For this review, take the finished solid that the model builds, in its own axes (mm). A direction names the side the tool comes from. Give positions to 0.01 mm unless a question says otherwise; leave off trailing zeros. Order: outer loops, then holes, each group sorted by start corner. A loop starts at its lowest first (then second) coordinate and runs counter-clockwise, first axis right, second up. Notation, with made-up numbers: M 14,8.25 L 43,8.25 A14 ccw 43,24.25 Z; hole C 86,24 d1. An arc over 180 degrees is marked long. Answer as CSV lines item,"result". Start each with the question number.
1. We need section C-C, the plane z = 13. Give the boundary of the cut face in (x, y).
2. Machinability: for faces 4 (the flat face through (-10.3, 20, 46)), 5 (the flat face through (10, 15, 63)), 6 (the flat face through (23, 9, 0)), 7 (the flat face through (0, 0, 11)), 8 (the flat face through (19.5, 9, 63)), which of the approach directions +Z, -Z, +X, -X, +Y, -Y give a long, thin tool a straight path to every point of the face, cutting with its end or side? Answer none if there is none.
3. For line 1 along X through (y, z) = (0.5, 11); line 2 along Z through (x, y) = (12.5, 9.25); line 3 along X through (y, z) = (10, 61), list the stretches that pass through material, from the lowest coordinate up.
4. Clearance check with flat-ended pins moving along their axes: P1, Ø3, axis at y = 12.5, z = 64.5, coming from the +X side; P2, Ø11, axis at y = 14.5, z = 67, coming from the -X side; P3, Ø1, axis at x = -0.5, z = 0.5, coming from the +Y side. State where each tip first meets the part, or that it passes through.
5. We need section D-D, the plane y = 2.5. Give the boundary of the cut face in (x, z), and give its area (3 significant figures).
6. We need section A-A, the plane x = 12.5. Give the boundary of the cut face in (y, z), and give its area (3 significant figures).
7. Mouldability with a two-part tool opening along Z and no side actions: class faces 1 (the flat face through (-19.5, 9, 63)), 2 (the flat face through (-20, 10, 0)), 3 (the flat face through (-21.274, 9.154, 32.86)) as pulls with the +Z half, pulls with the -Z half, needs draft (parallel to the pull), parting line crosses it, or undercut.
8. We need section B-B, the plane y = 11. Give the boundary of the cut face in (x, z), and give its area (3 significant figures).
from build123d import *

# Parameters (mm, degrees)
SKETCH1_W           = 46
SKETCH1_H           = 46
SKETCH1_W_2         = 40
SKETCH1_H_2         = 40
BOSS_EXTRUDE1_DEPTH = 20
SKETCH2_W           = 46
SKETCH2_H           = 46
BOSS_EXTRUDE2_DEPTH = 2
BOSS_EXTRUDE3_DEPTH = 22
CUT_EXTRUDE1_DEPTH  = 20
BOSS_EXTRUDE5_DEPTH = 2
BOSS_EXTRUDE6_DEPTH = 40
SKETCH8_R           = 2.55
CUT_EXTRUDE2_DEPTH  = 60
SKETCH9_W           = 1
SKETCH9_H           = 20
BOSS_EXTRUDE7_DEPTH = 40


with BuildPart() as part:
    # Sketch1 → Boss-Extrude1 (new body)
    with BuildSketch(Plane(origin=(0, 0, 0), x_dir=(1, 0, 0), z_dir=(0, 1, 0))):
        Rectangle(SKETCH1_W, SKETCH1_H)
        Rectangle(SKETCH1_W_2, SKETCH1_H_2, mode=Mode.SUBTRACT)
    extrude(amount=BOSS_EXTRUDE1_DEPTH)

    # Sketch2 → Boss-Extrude2 (add)
    with BuildSketch(Plane.XZ):
        Rectangle(SKETCH2_W, SKETCH2_H)
    extrude(amount=BOSS_EXTRUDE2_DEPTH)

    # Sketch3 → Boss-Extrude3 (add)
    with BuildSketch(Plane(origin=(0, 20, 0), x_dir=(1, 0, 0), z_dir=(0, 1, 0))):
        Polygon((-16, -43), (-19.47826087, -23), (-23, -23), (-19.5, -43), align=None)
        Polygon((23, -23), (19.47826087, -23), (16, -43), (19.5, -43), align=None)
    extrude(amount=-BOSS_EXTRUDE3_DEPTH)

    # Sketch3<3> → Cut-Extrude1 (cut)
    with BuildSketch(Plane(origin=(0, 20, 0), x_dir=(1, 0, 0), z_dir=(0, 1, 0))):
        Polygon((20, -20), (-20, -20), (-19.47826087, -23), (19.47826087, -23), align=None)
    extrude(amount=-CUT_EXTRUDE1_DEPTH, mode=Mode.SUBTRACT)

    # Sketch5 → Boss-Extrude5 (add)
    with BuildSketch(Plane.XZ.offset(2)):
        Polygon((-16, 43), (-19.47826087, 23), (19.47826087, 23), (16, 43), align=None)
    extrude(amount=-BOSS_EXTRUDE5_DEPTH)

    # Sketch6 → Boss-Extrude6 (add)
    with BuildSketch(Plane.XY.offset(43)):
        with BuildLine():
            Line((-10, 20), (-15, 20))
            Line((-15, 20), (-15, 0))
            Line((-15, 0), (-16, 0))
            Line((-16, 0), (-16, 20))
            Line((-16, 20), (-19.5, 20))
            Line((-19.5, 20), (-19.5, -2))
            Line((-19.5, -2), (19.5, -2))
            Line((19.5, -2), (19.5, 20))
            Line((19.5, 20), (16, 20))
            Line((16, 20), (16, 0))
            Line((16, 0), (15, 0))
            Line((15, 0), (15, 20))
            Line((15, 20), (10, 20))
            Line((10, 20), (10, 10))
            ThreePointArc((10, 10), (0, 0), (-10, 10))
            Line((-10, 10), (-10, 20))
        make_face()
    extrude(amount=BOSS_EXTRUDE6_DEPTH)

    # Sketch8 → Cut-Extrude2 (cut)
    with BuildSketch(Plane.XY.offset(83)):
        with Locations((-12.914377538, 14.827782421)):
            Circle(SKETCH8_R)
    extrude(amount=-CUT_EXTRUDE2_DEPTH, mode=Mode.SUBTRACT)

    # Sketch9 → Boss-Extrude7 (add)
    with BuildSketch(Plane.XY.offset(83)):
        with Locations((15.5, 10)):
            Rectangle(SKETCH9_W, SKETCH9_H)
        with BuildLine():
            Line((-15, 16.294983479), (-15, 20))
            Line((-15, 20), (-16, 20))
            Line((-16, 20), (-16, 0))
            Line((-16, 0), (-15, 0))
            Line((-15, 0), (-15, 13.360581363))
            ThreePointArc((-15, 13.360581363), (-15.464377538, 14.827782421), (-15, 16.294983479))
        make_face()
    extrude(amount=-BOSS_EXTRUDE7_DEPTH)


solid = part.part
Result set:
1,outline,"M -23,-2 L 23,-2 L 23,20 L 20,20 L 20,0 L -20,0 L -20,20 L -23,20 Z"
2,face 4,"+Z, -Z, +X, -X, +Y"
2,face 5,"+Z, +Y"
2,face 6,"+Z, -Z, +X, +Y, -Y"
2,face 7,"+Y"
2,face 8,"+Z, +X, +Y, -Y"
3,line 1,"-23 to -20, 20 to 23"
3,line 2,"-23 to -20, 43 to 83"
3,line 3,"-19.5 to -10, 10 to 19.5"
4,P1,"x = 19.5"
4,P2,"x = -19.5"
4,P3,"y = 0"
5,outline,"M -23,-23 L 23,-23 L 23,23 L 19.5,43 L 19.5,83 L 6.61,83 L 6.61,43 L 16,43 L 20,20 L 20,-20 L -20,-20 L -20,20 L -16,43 L -6.61,43 L -6.61,83 L -19.5,83 L -19.5,43 L -23,23 Z"
5,area,"1,570 mm2"
6,outline,"M -2,-23 L 20,-23 L 20,-20 L 0,-20 L 0,43 L 20,43 L 20,83 L -2,83 Z"
6,area,"1,070 mm2"
7,face 1,"needs draft"
7,face 2,"undercut"
7,face 3,"pulls with the +Z half"
8,outline,"M -23,-23 L 23,-23 L 23,23 L 19.5,43 L 19.5,83 L 10,83 L 10,43 L 16,43 L 20,20 L 20,-20 L -20,-20 L -20,20 L -16,43 L -10,43 L -10,83 L -19.5,83 L -19.5,43 L -23,23 Z"
8,area,"1,300 mm2"
